Autodesk Inventor part; units mm, degrees
ref_plane "YZ Plane" through (0, 0, 0) normal (1, 0, 0) x (0, 1, 0)
ref_plane "XZ Plane" through (0, 0, 0) normal (0, 1, 0) x (-1, 0, 0)
ref_plane "XY Plane" through (0, 0, 0) normal (0, 0, 1) x (1, 0, 0)
sketch "Sketch1" plane through (0, 0, 0) normal (0, 0, 1) x (1, 0, 0)
  line L0 (0, 0) -> (110, 0) construction
  line L1 (110, 0) -> (110, 65) construction
  line L2 (110, 65) -> (0, 65) construction
  line L3 (0, 65) -> (0, 0) construction
  circle A0 centre (0, 65) radius 1.5
  circle A1 centre (0, 0) radius 1.5
  circle A2 centre (110, 0) radius 1.5
  circle A3 centre (110, 65) radius 1.5
  line L4 (-7.5, 72.5) -> (7.5, 72.5)
  line L5 (7.5, 72.5) -> (7.5, -7.5)
  line L6 (7.5, -7.5) -> (-7.5, -7.5)
  line L7 (-7.5, -7.5) -> (-7.5, 72.5)
  line L8 (102.5, 72.5) -> (117.5, 72.5)
  line L9 (117.5, 72.5) -> (117.5, -7.5)
  line L10 (117.5, -7.5) -> (102.5, -7.5)
  line L11 (102.5, -7.5) -> (102.5, 72.5)
  point P0 (7.5, 32.5)
  point P1 (0, 32.5)
  point P2 (102.5, 32.5)
  point P3 (110, 32.5)
  point P4 (0, 72.5)
  point P5 (110, 72.5)
  dimension "d0" = 110
  dimension "d1" = 65
  dimension "d2" = 3
  dimension "d3" = 3
  dimension "d4" = 3
  dimension "d5" = 3
  dimension "d6" = 15
  dimension "d7" = 15
  dimension "d8" = 80
extrude "Extrusion1" add sketch "Sketch1" along normal blind 22
sketch "Sketch2" plane through (0, 0, 22) normal (0, 0, 1) x (1, 0, 0)
  circle A0 centre (0, 65) radius 1.5
  circle A1 centre (0, 0) radius 1.5
  circle A2 centre (110, 0) radius 1.5
  circle A3 centre (110, 65) radius 1.5
  line L0 (-7.5, 72.5) -> (-7.5, -7.5)
  line L1 (7.5, 72.5) -> (-7.5, 72.5)
  line L2 (102.5, -7.5) -> (117.5, -7.5)
  line L3 (117.5, -7.5) -> (117.5, 72.5)
  line L4 (-7.5, 72.5) -> (117.5, 72.5)
  line L5 (117.5, 72.5) -> (117.5, -7.5)
  line L6 (117.5, -7.5) -> (-7.5, -7.5)
  line L7 (-7.5, -7.5) -> (-7.5, 72.5)
extrude "Extrusion2" add sketch "Sketch2" along normal blind 3
sketch "Sketch3" plane through (0, 0, 25) normal (0, 0, 1) x (1, 0, 0)
  circle A0 centre (0, 65) radius 1.5
  circle A1 centre (110, 65) radius 1.5
  circle A2 centre (110, 0) radius 1.5
  circle A3 centre (0, 0) radius 1.5
  circle A4 centre (0, 65) radius 1.5
  circle A5 centre (0, 65) radius 4
  circle A6 centre (0, 0) radius 1.5
  circle A7 centre (0, 0) radius 4
  circle A8 centre (110, 0) radius 1.5
  circle A9 centre (110, 0) radius 4
  circle A10 centre (110, 65) radius 4
  dimension "d13" = 8
  dimension "d14" = 8
  dimension "d15" = 8
  dimension "d16" = 8
extrude "Extrusion3" cut sketch "Sketch3" against normal blind 20 contours A0 | A1 | A2 | A3 | A5 | A7 | A9 | A10
properties part number "BP010" material "ABS Plastic"
Design review of the part built by this model. Coordinates are the model's own, in mm. A direction names the side the tool comes from. Coordinates: 2 decimals unless noted, no trailing zeros. Write each loop counter-clockwise with the first axis right and the second up, starting at its lowest first coordinate (ties: lowest second). Pieces come first, ordered by that corner, then holes. Notation, with made-up numbers: M 6.5,1.5 L 28.5,1.5 A19 ccw 28.5,32.5 Z; hole C 74,8.5 d6. An arc over 180 degrees is marked long. Answer as a JSON object with one key per item and string values.
Item 1: Add section B-B, the plane z = 10.5. Give the boundary of the cut face in (x, y), and give its area (3 significant figures).
Outcome:
{"outline": "M -7.5,-7.5 L 7.5,-7.5 L 7.5,72.5 L -7.5,72.5 Z; M 102.5,-7.5 L 117.5,-7.5 L 117.5,72.5 L 102.5,72.5 Z; hole C 0,0 d8; hole C 0,65 d8; hole C 110,0 d8; hole C 110,65 d8", "area": "2,200 mm²"}
Item 2: Add section A-A, the plane y = 0. Give the boundary of the cut face in (x, z).
Outcome:
{"outline": "M -7.5,0 L -1.5,0 L -1.5,5 L -4,5 L -4,25 L -7.5,25 Z; M 1.5,0 L 7.5,0 L 7.5,22 L 102.5,22 L 102.5,0 L 108.5,0 L 108.5,5 L 106,5 L 106,25 L 4,25 L 4,5 L 1.5,5 Z; M 111.5,0 L 117.5,0 L 117.5,25 L 114,25 L 114,5 L 111.5,5 Z"}
Item 3: Add section C-C, the plane x = 0. Give the boundary of the cut face in (y, z), and give its area (3 significant figures).
Outcome:
{"outline": "M -7.5,0 L -1.5,0 L -1.5,5 L -4,5 L -4,25 L -7.5,25 Z; M 1.5,0 L 63.5,0 L 63.5,5 L 61,5 L 61,25 L 4,25 L 4,5 L 1.5,5 Z; M 66.5,0 L 72.5,0 L 72.5,25 L 69,25 L 69,5 L 66.5,5 Z", "area": "1,650 mm²"}
Item 4: Insertion check: pin 1 Ø6.5 at (x, y) = (110, 65) entering from +Z; pin 2 Ø3 at (x, y) = (39, 22) entering from -Z. Each pin has a flat end and moves straight along its axis. Give the tip position at first contact, or say it passes through.
Outcome:
{"pin 1": "z = 5", "pin 2": "z = 22"}
Item 5: Draft analysis for pull direction X (two halves, no side actions). For faces 1 (the flat face through (110, 33, 0)), 2 (the flat face through (117.5, 32, 12)), 3 (the cylindrical face through (-1.5, -0.07, 2.46)), 4 (the cylindrical face through (-0.867, 61.095, 15.14)), state which applies: pulls with the +X half, pulls with the -X half, needs draft (parallel to the pull), parting line crosses it, or undercut.
Outcome:
{"face 1": "needs draft", "face 2": "pulls with the +X half", "face 3": "undercut", "face 4": "undercut"}
Item 6: Wall thickness on probe 1 along X at (y, z) = (65, 1); probe 2 along Y at (x, z) = (0, 11.25); probe 3 along Y at (x, z) = (110, 2.4): over which ranges is each line inside the solid? List them lowest first.
Outcome:
{"probe 1": "-7.5 to -1.5, 1.5 to 7.5, 102.5 to 108.5, 111.5 to 117.5", "probe 2": "-7.5 to -4, 4 to 61, 69 to 72.5", "probe 3": "-7.5 to -1.5, 1.5 to 63.5, 66.5 to 72.5"}
Item 7: Machinability: for faces 5 (the flat face through (0, 33, 0)), 6 (the flat face through (54, 33, 22)), 7 (the cylindrical face through (-0.867, -3.905, 15.14)), which of the approach directions +Z, -Z, +X, -X, +Y, -Y give a long, thin tool a straight path to every point of the face, cutting with its end or side? Answer none if there is none.
Outcome:
{"face 5": "-Z, +X, -X, +Y, -Y", "face 6": "-Z, +Y, -Y", "face 7": "+Z"}
Item 8: Add section D-D, the plane y = 41. Give the boundary of the cut face in (x, z).
Outcome:
{"outline": "M -7.5,0 L 7.5,0 L 7.5,22 L 102.5,22 L 102.5,0 L 117.5,0 L 117.5,25 L -7.5,25 Z"}
